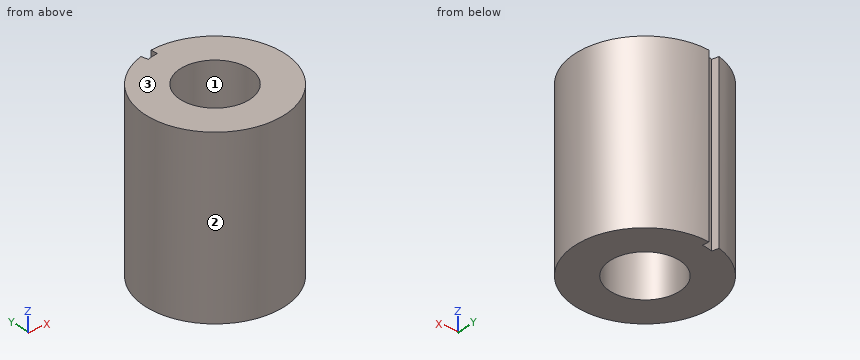
```python
from build123d import *

# Parameters (mm, degrees)
SKETCH1_R           = 4
SKETCH1_R_2         = 2
BOSS_EXTRUDE1_DEPTH = 10
CUT_EXTRUDE1_DEPTH  = 11


with BuildPart() as part:
    # Sketch1 → Boss-Extrude1 (new body)
    with BuildSketch(Plane.XY):
        Circle(SKETCH1_R)
        Circle(SKETCH1_R_2, mode=Mode.SUBTRACT)
    extrude(amount=BOSS_EXTRUDE1_DEPTH)

    # Sketch2 → Cut-Extrude1 (cut)
    with BuildSketch(Plane.XY.offset(10)):
        with BuildLine():
            Line((-0.961093553, 3.469336995), (-1.43156592, 5.16763908))
            ThreePointArc((-1.43156592, 5.16763908), (-0.975728957, 5.272743844), (-0.512466108, 5.337719844))
            Line((-0.512466108, 5.337719844), (-0.344048336, 3.583522114))
            ThreePointArc((-0.344048336, 3.583522114), (-0.65506366, 3.539899942), (-0.961093553, 3.469336995))
        make_face()
    extrude(amount=-CUT_EXTRUDE1_DEPTH, mode=Mode.SUBTRACT)


solid = part.part
```
Here's how the part is built. I have some questions about the finished solid (model axes, mm). Face numbers are marked on the shaded views. Round coordinates to 2 decimals unless told otherwise and drop trailing zeros. Loops run counter-clockwise (first coordinate to the right, second up) from the corner with the lowest first, then second, coordinate; pieces in that order, holes last.
1. Suppose I cut it at C-C, the plane z = 4. Please give me the cut outline in (x, y), and give its area (3 significant figures).
Answers:
outline: (-1.07, 3.85) arc R4 ccw (long way) to (-0.38, 3.98) - (-0.34, 3.58) arc R3.6 ccw to (-0.96, 3.47) - close; hole circle Ø4 at (0, 0)
area: 37.4 mm2
2. Suppose I cut it at D-D, the plane y = -3.5. Please give me the cut outline in (x, z), and give its area (3 significant figures).
Answers:
outline: (-1.94, 0) - (1.94, 0) - (1.94, 10) - (-1.94, 10) - close
area: 38.7 mm2
3. Suppose I cut it at A-A, the plane y = 0. Please give me the cut outline in (x, z).
Answers:
outline: (-4, 0) - (-2, 0) - (-2, 10) - (-4, 10) - close; (2, 0) - (4, 0) - (4, 10) - (2, 10) - close
4. Thinking about a two-plate mould opening in X: for the marked faces 1, 2 and 3, which applies, released by +X, released by -X, zero draft, split by the parting line, or undercut?
Answers:
face 1: undercut
face 2: split by the parting line
face 3: zero draft
5. Will these pins go through, and if not, where does the flat tip stop? pin 1 (3.5 mm diameter, centred on x = 0, y = 0, fed in from +Z); pin 2 (3 mm diameter, centred on x = -3, z = 5, fed in from +Y); pin 3 (2 mm diameter, centred on x = 2, z = 3.5, fed in from +Y).
Answers:
pin 1: passes through
pin 2: stops at y = 3.71
pin 3: stops at y = 3.87
6. If I drill on probe 1 along Y at (x, z) = (0, 6.5); probe 2 along Y at (x, z) = (-0.5, 5); probe 3 along X at (y, z) = (-3, 8.75), over which ranges is the centre line in solid material (lowest first)?
Answers:
probe 1: y = -4 to -2, 2 to 4
probe 2: y = -3.97 to -1.94, 1.94 to 3.57
probe 3: x = -2.65 to 2.65
